Design review of the part built by this model. Coordinates are the model's own, in mm. Face numbers are marked on the shaded views. Coordinates: 2 decimals unless noted, no trailing zeros. Loops run counter-clockwise (first coordinate to the right, second up) from the corner with the lowest first, then second, coordinate; pieces in that order, holes last.
Q1. Add section C-C on z = -1.5. Give the boundary of the cut face in (x, y).
Q2. Draft analysis for pull direction X (two halves, no side actions). For the marked faces 1 and 2, state which applies: released by +X, released by -X, zero draft, split by the parting line, or undercut.
Q3. For P1, Ø1, axis at y = 129.5, z = 16, coming from the +X side; P2, Ø3, axis at x = 94.5, y = 136.5, coming from the -Z side; P3, Ø3.5, axis at y = 131.5, z = -18.5, coming from the -X side; P4, Ø12, axis at x = 87, z = -17, coming from the -Y side, all flat-tipped, find the tip position at first contact; note any pin that passes through.
Q4. Wall thickness on probe 1 along Z at (x, y) = (96.5, 164.5); probe 2 along X at (y, z) = (75, 16.5); probe 3 along Z at (x, y) = (87, 72): over which ranges is each line inside the solid? List them lowest first.
Q5. Add section A-A on x = 89.5. Give the boundary of the cut face in (y, z), and give its area (3 significant figures).
```python
from build123d import *

# Parameters (mm, degrees)
BOSS_EXTRUDE1_DEPTH = 22.225
SKETCH4_W           = 42.895640362
SKETCH4_H           = 166.52307566
CUT_EXTRUDE2_DEPTH  = 22.225
CIRPATTERN1_COUNT   = 4
SKETCH5_R           = 4.7625
CUT_EXTRUDE3_DEPTH  = 190.365652901


with BuildPart() as part:
    # Sketch1 → Boss-Extrude1 (new body)
    with BuildSketch(Plane.XY):
        Polygon((75.93611291, 50.130135743), (91.347997502, 50.130135743), (91.347997502, 200.018674704), (69.122997502, 200.018674704), align=None)
    boss_extrude1 = extrude(amount=BOSS_EXTRUDE1_DEPTH)

    # Sketch4 → Cut-Extrude2 (cut)
    with BuildSketch(Plane(origin=(39.013250999, 1.751956449, -39.013250999), x_dir=(0.7060390157604001, 0.031705883905462015, 0.7074628224506635), z_dir=(-0.7067505605587739, -0.03173783703590832, 0.7067505605587739))):
        with Locations((68.323098286, 123.218808293)):
            Rectangle(SKETCH4_W, SKETCH4_H)
    cut_extrude2 = extrude(amount=CUT_EXTRUDE2_DEPTH, mode=Mode.SUBTRACT)

    # CirPattern1: Boss-Extrude1, Cut-Extrude2 ×4 about axis
    cirpattern1_axis = Axis((91.347997502, 0, 0), (0, 1, 0))
    add([boss_extrude1.rotate(cirpattern1_axis, i * 360 / CIRPATTERN1_COUNT) for i in range(1, CIRPATTERN1_COUNT)])
    add([cut_extrude2.rotate(cirpattern1_axis, i * 360 / CIRPATTERN1_COUNT) for i in range(1, CIRPATTERN1_COUNT)], mode=Mode.SUBTRACT)

    # Sketch5 → Cut-Extrude3 (cut, through all)
    with BuildSketch(Plane(origin=(0, 200.018674704, 0), x_dir=(1, 0, 0), z_dir=(0, 1, 0))):
        with Locations(Location((91.347997502, 0, 0), (0, 0, 270))):
            Circle(SKETCH5_R)
    extrude(amount=-CUT_EXTRUDE3_DEPTH, mode=Mode.SUBTRACT)


solid = part.part
```
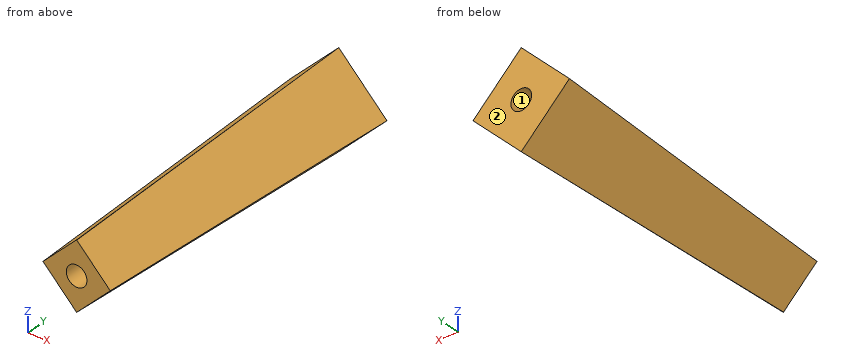
Entries:
1. outline: (70.62, 200.02) - (77.35, 50.13) - (86.83, 50.13) - (86.83, 200.02) - close; (95.87, 50.13) - (105.34, 50.13) - (112.07, 200.02) - (95.87, 200.02) - close
2. face 1: undercut
2. face 2: zero draft
3. P1: stops at x = 94.91
3. P2: stops at z = -17.72
3. P3: stops at x = 88.95
3. P4: stops at y = 50.13
4. probe 1: z = -15.48 to 15.48
4. probe 2: x = 91.24 to 91.46
4. probe 3: z = -12.13 to -1.94, 1.94 to 12.13
5. outline: (50.13, -13.65) - (200.02, -20.38) - (200.02, -4.39) - (50.13, -4.39) - close; (50.13, 4.39) - (200.02, 4.39) - (200.02, 20.38) - (50.13, 13.65) - close
5. area: 3,780 mm2
